Model file for the job. Use its own axes, mm. A direction names the side the tool comes from. Coordinates: 2 decimals unless noted, no trailing zeros.
from build123d import *

# Parameters (mm, degrees)
SKETCH4_R                  = 34.925
SKETCH4_R_2                = 18.161
BOSS_EXTRUDE1_DEPTH        = 72.771
CUT_EXTRUDE2_REACH         = 137.172
CUT_EXTRUDE2_START         = 21.75002
TRIPOD_WALLS_R             = 3.175
BOLT_HOLE_FACE_R           = 3.175
SKETCH12_R                 = 3.175
CUT_EXTRUDE3_DEPTH         = 63.5
CUT_EXTRUDE4_START         = -22.44598
SKETCH13_R                 = 34.925
CUT_EXTRUDE4_DEPTH         = 22.44598
SKETCH16_R                 = 22.86
COMPENSATING_SPACING_DEPTH = 1.016
F_1_4_0_2500_DOWEL_HOLE1_D = 6.35
BOLT_CIRCLE_PATTERN_2_R    = 4.1021
F_5_16_CLEARNCE_DEPTH      = 13.716


with BuildPart() as part:
    # Sketch2 → Revolve1 (revolve)
    with BuildSketch(Plane.XY, mode=Mode.PRIVATE) as revolve1_sk:
        Polygon((0, 0), (0, -30.9499), (12.7, -30.9499), (12.7, 0), (3.2004, 0), (3.2004, -1.5621), (1.27, -1.5621), (1.27, 0), align=None)
    revolve(revolve1_sk.sketch.rotate(Axis((11.964521893, -30.9499, 0), (-1, 0, 0)), 90), axis=Axis((11.964521893, -30.9499, 0), (-1, 0, 0)))

    # Sketch4 → Boss-Extrude1 (add)
    with BuildSketch(Plane(origin=(12.7, 0, 0), x_dir=(0, 0, -1), z_dir=(1, 0, 0))):
        with Locations((0, -30.9499)):
            Circle(SKETCH4_R)
        with Locations((0, -30.9499)):
            Circle(SKETCH4_R_2, mode=Mode.SUBTRACT)
    extrude(amount=BOSS_EXTRUDE1_DEPTH)

    # Sketch5 → Cut-Extrude2 (cut, up to next)
    with BuildSketch(Plane(origin=(0, 0, 0), x_dir=(0, 0, -1), z_dir=(1, 0, 0)).offset(CUT_EXTRUDE2_START), mode=Mode.PRIVATE) as cut_extrude2_sk1:
        with BuildLine():
            ThreePointArc((-11.141810341, -4.2233215), (0, -23.4823), (11.141810341, -4.2233215))
            ThreePointArc((11.141810341, -4.2233215), (0, -1.9939), (-11.141810341, -4.2233215))
        make_face()
    cut_extrude2_tool1 = extrude(cut_extrude2_sk1.sketch, amount=CUT_EXTRUDE2_REACH, mode=Mode.PRIVATE) & part.part
    # Sketch5 → Cut-Extrude2 (cut, up to next)
    with BuildSketch(Plane(origin=(0, 0, 0), x_dir=(0, 0, -1), z_dir=(1, 0, 0)).offset(CUT_EXTRUDE2_START), mode=Mode.PRIVATE) as cut_extrude2_sk2:
        with BuildLine():
            ThreePointArc((-28.716801071, -34.664098733), (-25.076631449, -45.427900247), (-17.57499054, -53.962280223))
            ThreePointArc((-17.57499054, -53.962280223), (-6.467131268, -34.683700064), (-28.716801071, -34.664098733))
        make_face()
    cut_extrude2_tool2 = extrude(cut_extrude2_sk2.sketch, amount=CUT_EXTRUDE2_REACH, mode=Mode.PRIVATE) & part.part
    # Sketch5 → Cut-Extrude2 (cut, up to next)
    with BuildSketch(Plane(origin=(0, 0, 0), x_dir=(0, 0, -1), z_dir=(1, 0, 0)).offset(CUT_EXTRUDE2_START), mode=Mode.PRIVATE) as cut_extrude2_sk3:
        with BuildLine():
            ThreePointArc((28.716801071, -34.664098733), (6.467131268, -34.683700064), (17.57499054, -53.962280223))
            ThreePointArc((17.57499054, -53.962280223), (25.076631449, -45.427900247), (28.716801071, -34.664098733))
        make_face()
    cut_extrude2_tool3 = extrude(cut_extrude2_sk3.sketch, amount=CUT_EXTRUDE2_REACH, mode=Mode.PRIVATE) & part.part
    add(cut_extrude2_tool1.solids().sort_by_distance((21.75002, -12.135894, 0))[0], mode=Mode.SUBTRACT)
    add(cut_extrude2_tool2.solids().sort_by_distance((21.75002, -40.356903, 16.293407))[0], mode=Mode.SUBTRACT)
    add(cut_extrude2_tool3.solids().sort_by_distance((21.75002, -40.356903, -16.293407))[0], mode=Mode.SUBTRACT)

    # Tripod walls
    tripod_walls_edges = [part.edges().sort_by_distance(p)[0] for p in [
        (53.61051, -4.2233215, 11.141810341),
        (53.61051, -4.2233215, -11.141810341),
        (53.61051, -53.962280223, 17.57499054),
        (53.61051, -34.664098733, 28.716801071),
        (53.61051, -34.664098733, -28.716801071),
        (53.61051, -53.962280223, -17.57499054),
    ]]
    fillet(tripod_walls_edges, radius=TRIPOD_WALLS_R)

    # Bolt Hole Face
    bolt_hole_face_edges = [part.edges().sort_by_distance(p)[0] for p in [
        (12.7, -30.9499, 18.161),
    ]]
    fillet(bolt_hole_face_edges, radius=BOLT_HOLE_FACE_R)

    # Sketch12 → Cut-Extrude3 (cut)
    with BuildSketch(Plane(origin=(85.471, 0, 0), x_dir=(0, 0, -1), z_dir=(1, 0, 0))):
        with Locations((-21.997045256, -18.2499)):
            Circle(SKETCH12_R)
        with Locations((21.997045256, -18.2499)):
            Circle(SKETCH12_R)
        with Locations((0, -56.3499)):
            Circle(SKETCH12_R)
    extrude(amount=-CUT_EXTRUDE3_DEPTH, mode=Mode.SUBTRACT)

    # Sketch13 → Cut-Extrude4 (cut)
    with BuildSketch(Plane(origin=(85.471, 0, 0), x_dir=(0, 0, -1), z_dir=(1, 0, 0)).offset(CUT_EXTRUDE4_START)):
        with Locations((0, -30.9499)):
            Circle(SKETCH13_R)
    extrude(amount=CUT_EXTRUDE4_DEPTH, mode=Mode.SUBTRACT)

    # Sketch16 → Compensating Spacing (add)
    with BuildSketch(Plane.ZY):
        with Locations(Location((0, -30.9499, 0), (0, 0, 270))):
            Circle(SKETCH16_R)
    extrude(amount=COMPENSATING_SPACING_DEPTH)

    # 1/4 (0.2500) Dowel Hole1 (through all)
    with Locations(Plane(origin=(12.7, 0, 0), x_dir=(0, 0, -1), z_dir=(1, 0, 0))):
        with Locations((0, -21.4249), (9.525, -30.9499), (0, -40.4749), (-9.525, -30.9499)):
            Hole(F_1_4_0_2500_DOWEL_HOLE1_D / 2)

    # Bolt Circle Pattern<2> → 5/16 Clearnce (cut)
    with BuildSketch(Plane(origin=(12.7, 0, 0), x_dir=(0, 0, -1), z_dir=(1, 0, 0))):
        with Locations((0, -30.9499)):
            Circle(BOLT_CIRCLE_PATTERN_2_R)
    extrude(amount=-F_5_16_CLEARNCE_DEPTH, mode=Mode.SUBTRACT)


solid = part.part
Q1. Mould opens along Z. For faces 1 (the face through (-1.016, -36, 0)), 2 (the face through (2.222, -60.088, 3.826)), 3 (the face through (21.971, -56, 0)) say: pulls with the +Z half, pulls with the -Z half, needs draft (parallel to the pull), parting line crosses it, or undercut.
Established:
face 1: needs draft
face 2: parting line crosses it
face 3: undercut
Q2. Cut at A-A, the plane z = 0. Count the separate pieces of the cut face and the enclosed holes in it, plus the area to 3 significant figures.
Established:
separate pieces: 4
enclosed holes: 0
area: 1,530 mm2
Q3. Probe line 1 (Y direction, x = 33, z = -23); line 2 (Z direction, x = 59, y = -10); line 3 (Y direction, x = 30.5, z = -22.5). List the from-to ranges inside material, lowest first.
Established:
line 1: y = -57.23 to -48.54, -29.45 to -21.26, -15.24 to -4.67
line 2: z = -27.94 to -12.84, 12.84 to 27.94
line 3: y = -57.66 to -49.18, -29.23 to -21.38, -15.11 to -4.24
Q4. Which spindle directions (+Z, -Z, +X, -X, +Y, -Y) get a long thin tool onto all of the face, cutting with end or side? Do faces 4 (the face through (0.626, -0.736, 6.709)), 5 (the face through (42.785, -19.466, 19.064)), 6 (the face through (5.746, -29.996, 12.553)). Say none if no direction does.
Established:
face 4: -X
face 5: +X
face 6: +X, -X
Q5. Drop flat-ended pins along their axis: P1, Ø5.5, axis at y = -30.95, z = -9.52, coming from the -X side; P2, Ø10, axis at x = 27, z = 25, coming from the -Y side; P3, Ø8, axis at x = 12, y = -46.5, coming from the +Z side; P4, Ø5, axis at x = 8, z = -27, coming from the +Y side. Give the stop position or say it passes through.
Established:
P1: passes through
P2: stops at y = -59.58
P3: stops at z = 32.94
P4: stops at y = -12.04
